Source: CAD feature listing. Evaluate the final solid. Frame: model axes, mm. Coordinates: 2 decimals unless noted, no trailing zeros. Loops run counter-clockwise (first coordinate to the right, second up) from the corner with the lowest first, then second, coordinate; pieces in that order, holes last.
Item 1: Section query D-D, the plane y = 64. Return the cut outline in (x, z).
Item 2: Section query B-B, the plane z = 75. Return the cut outline in (x, y).
Item 3: Pull-direction query (Z, two-part tool) for faces 1 (the cylindrical face through (-2.465, 227.889, 525.275)), 2 (the flat face through (-5, 253, 294)); classes: +Z half, -Z half, draft (parallel to the pull), parting line (faces both ways), or undercut.
Item 4: Section query C-C, the plane x = -3.6. State how many separate pieces and enclosed holes the cut face has, then the cut area to 3 significant figures.
Item 5: Line query: probe 1 along Z at (x, y) = (-4.35, 424); probe 2 along Y at (x, z) = (-3.55, 505.5); probe 3 along Z at (x, y) = (-1.25, 226.5). Output: solid intervals per line, ascending.
Item 6: Section query A-A, the plane y = 250. Return the cut outline in (x, z), then the cut area to 3 significant figures.
```python
from build123d import *

# Parameters (mm, degrees)
PAD_DEPTH    = 5
SKETCH002_R  = 30
POCKET_DEPTH = 5.001


with BuildPart() as part:
    # Sketch → Pad (new body)
    with BuildSketch(Plane.YZ):
        Polygon((0, 0), (0, 580), (500, 580), (500, 0), (250, 0), align=None)
    extrude(amount=-PAD_DEPTH)

    # Sketch002 (on Face6 of Pad) → Pocket (cut, through all)
    with BuildSketch(Plane.YZ):
        with Locations((250, 505)):
            Circle(SKETCH002_R)
        with Locations((250, 75)):
            Circle(SKETCH002_R)
        with Locations((75.351784, 505)):
            Circle(SKETCH002_R)
        with Locations((75.351784, 75)):
            Circle(SKETCH002_R)
        with Locations((162.675892, 75)):
            Circle(SKETCH002_R)
        with Locations((337.324108, 75)):
            Circle(SKETCH002_R)
        with Locations((424.648216, 75)):
            Circle(SKETCH002_R)
        with Locations((424.648216, 505)):
            Circle(SKETCH002_R)
        with Locations((337.324108, 505)):
            Circle(SKETCH002_R)
        with Locations((162.675892, 505)):
            Circle(SKETCH002_R)
    extrude(amount=-POCKET_DEPTH, mode=Mode.SUBTRACT)


solid = part.part
```
Verdict:
1. outline: (-5, 0) - (0, 0) - (0, 47.23) - (-5, 47.23) - close; (-5, 102.77) - (0, 102.77) - (0, 477.23) - (-5, 477.23) - close; (-5, 532.77) - (0, 532.77) - (0, 580) - (-5, 580) - close
2. outline: (-5, 0) - (0, 0) - (0, 45.35) - (-5, 45.35) - close; (-5, 105.35) - (0, 105.35) - (0, 132.68) - (-5, 132.68) - close; (-5, 192.68) - (0, 192.68) - (0, 220) - (-5, 220) - close; (-5, 280) - (0, 280) - (0, 307.32) - (-5, 307.32) - close; (-5, 367.32) - (0, 367.32) - (0, 394.65) - (-5, 394.65) - close; (-5, 454.65) - (0, 454.65) - (0, 500) - (-5, 500) - close
3. face 1: undercut
3. face 2: draft
4. separate pieces: 1
4. enclosed holes: 10
4. area: 262,000 mm2
5. probe 1: z = 0 to 45.01, 104.99 to 475.01, 534.99 to 580
5. probe 2: y = 0 to 45.36, 105.35 to 132.68, 192.67 to 220, 280 to 307.33, 367.32 to 394.65, 454.64 to 500
5. probe 3: z = 0 to 56.35, 93.65 to 486.35, 523.65 to 580
6. outline: (-5, 0) - (0, 0) - (0, 45) - (-5, 45) - close; (-5, 105) - (0, 105) - (0, 475) - (-5, 475) - close; (-5, 535) - (0, 535) - (0, 580) - (-5, 580) - close
6. area: 2,300 mm2
